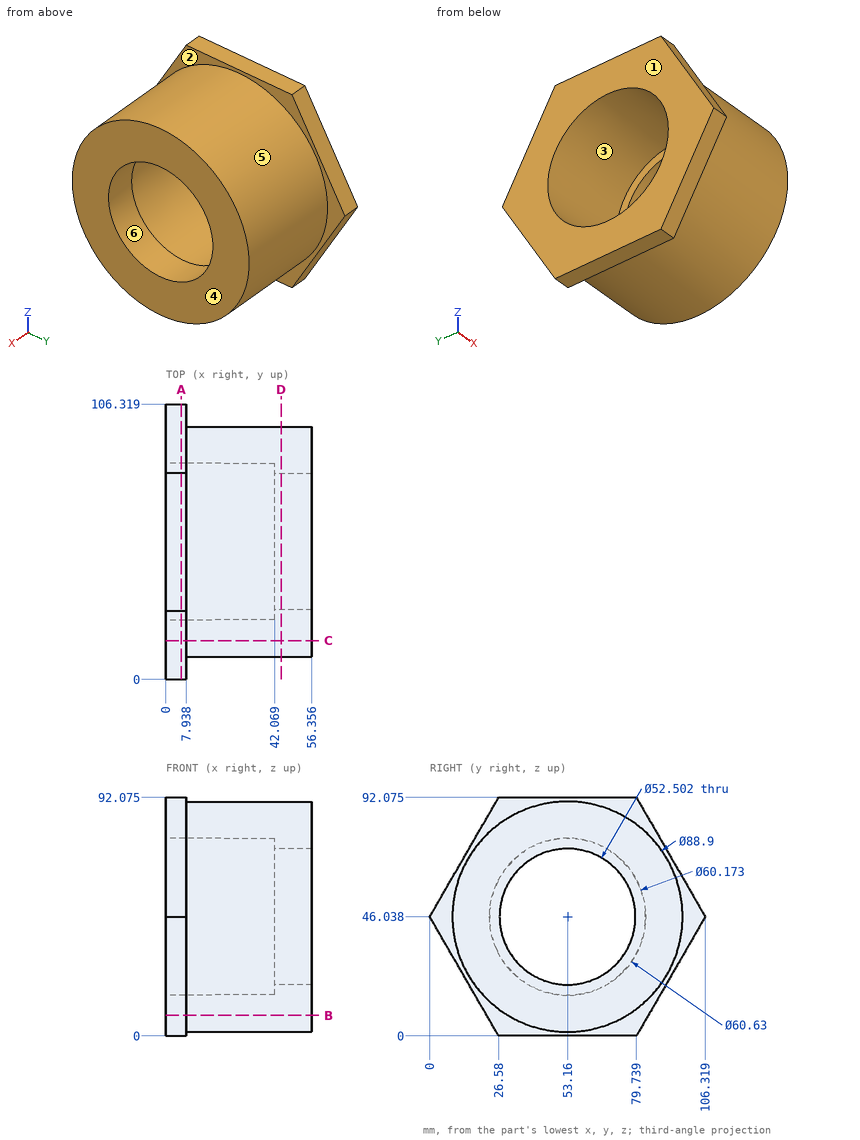
Could you check a few things on this drawing? It's one solid part, dimensions in mm from its lowest x, y, z. A direction names the side the tool comes from. Round coordinates to 2 decimals unless told otherwise and drop trailing zeros. Write each loop counter-clockwise with the first axis right and the second up, starting at its lowest first coordinate (ties: lowest second). Pieces come first, ordered by that corner, then holes. Notation, with made-up numbers: M 6.5,-8.75 L 25.5,-8.75 A27 ccw 25.5,15.25 Z; hole C -30,21.25 d10. An arc over 180 degrees is marked long. Answer as CSV lines item,"result". Start each with the question number.
1. Suppose I cut it at C-C on y = 15. Write out the boundary of the cut face in (x, z).
2. Suppose I cut it at D-D on x = 44.5. Write out the boundary of the cut face in (y, z), then the cut area to 3 significant figures.
3. Suppose I cut it at B-B on z = 8. Write out the boundary of the cut face in (x, y).
4. I need wall thicknesses on probe 1 along Y at (x, z) = (13.5, 47.5) (1 decimal); probe 2 along X at (y, z) = (55, 72.5); probe 3 along Y at (x, z) = (15, 43.5). Which ranges of each line are inside material? Lowest first, please.
5. I'm going to push flat-ended pins straight in: pin 1 Ø1.5 at (x, y) = (21, 68.5) entering from -Z; pin 2 Ø8 at (x, y) = (49, 44.5) entering from -Z; pin 3 Ø2 at (x, y) = (11.5, 33) entering from -Z. Where does each tip first touch, or does it pass through?
6. Suppose I cut it at A-A on x = 6. Write out the boundary of the cut face in (y, z) (1 decimal), then the cut area to 3 significant figures.
7. On a 3-axis mill with a long thin cutter (end or side, diameter ignored), from which of +Z, -Z, +X, -X, +Y, -Y can I reach the whole of each face in a straight line? I mean the marked faces 1 and 2. Say none if no direction works.
8. Thinking about a two-plate mould opening in Y: for the marked faces 3, 4, 5 and 6, which applies, released by +Y, released by -Y, zero draft, split by the parting line, or undercut?
Check result:
1,outline,"M 0,20.06 L 7.94,20.06 L 7.94,23.24 L 56.36,23.24 L 56.36,68.83 L 7.94,68.83 L 7.94,72.02 L 0,72.02 Z"
2,outline,"C 53.16,46.04 d88.9; hole C 53.16,46.04 d52.5"
2,area,"4,040 mm2"
3,outline,"M 0,21.96 L 7.94,21.96 L 7.94,30.16 L 56.36,30.16 L 56.36,76.16 L 7.94,76.16 L 7.94,84.36 L 0,84.36 Z"
4,probe 1,"y = 8.7 to 23, 83.4 to 97.6"
4,probe 2,"x = 42.07 to 56.36"
4,probe 3,"y = 8.78 to 23.03, 83.29 to 97.54"
5,pin 1,"stops at z = 4.05"
5,pin 2,"stops at z = 1.83"
5,pin 3,"stops at z = 5.93"
6,outline,"M 0,46 L 26.6,0 L 79.7,0 L 106.3,46 L 79.7,92.1 L 26.6,92.1 Z; hole C 53.2,46 d60.6"
6,area,"4,460 mm2"
7,face 1,"+Z, -Z, -X, +Y, -Y"
7,face 2,"+X"
8,face 3,"undercut"
8,face 4,"zero draft"
8,face 5,"split by the parting line"
8,face 6,"undercut"
